Check sheet for the modelled part. Datum: model origin and axes. Units: mm. A direction names the side the tool comes from. Round coordinates to 2 decimals unless told otherwise and drop trailing zeros. Write each loop counter-clockwise with the first axis right and the second up, starting at its lowest first coordinate (ties: lowest second). Pieces come first, ordered by that corner, then holes. Notation, with made-up numbers: M 31,1 L 79,1 A11 cw 79,18 Z; hole C 74.25,79.25 d4. An arc over 180 degrees is marked long. One line per item, written item: value.
from build123d import *

# Parameters (mm, degrees)
SKETCH1_W           = 640
SKETCH1_H           = 50
BOSS_EXTRUDE1_DEPTH = 10
SKETCH2_W           = 15
SKETCH2_H           = 50
BOSS_EXTRUDE2_DEPTH = 10
SKETCH3_W           = 610
SKETCH3_H           = 20
CUT_EXTRUDE1_DEPTH  = 10


with BuildPart() as part:
    # Sketch1 → Boss-Extrude1 (new body)
    with BuildSketch(Plane.XY):
        with Locations((-320, -120.36)):
            Rectangle(SKETCH1_W, SKETCH1_H)
    extrude(amount=BOSS_EXTRUDE1_DEPTH)

    # Sketch2 → Boss-Extrude2 (add)
    with BuildSketch(Plane.XY):
        with Locations((-160, -70.36)):
            Rectangle(SKETCH2_W, SKETCH2_H)
        with Locations((-480, -70.36)):
            Rectangle(SKETCH2_W, SKETCH2_H)
    extrude(amount=BOSS_EXTRUDE2_DEPTH)

    # Sketch3 → Cut-Extrude1 (cut)
    with BuildSketch(Plane(origin=(0, 0, 0), x_dir=(-1, 0, 0), z_dir=(0, 0, -1))):
        with Locations((320, -120.36)):
            Rectangle(SKETCH3_W, SKETCH3_H)
    extrude(amount=-CUT_EXTRUDE1_DEPTH, mode=Mode.SUBTRACT)


solid = part.part
Q1. Draft check along Y on faces 1 (the flat face through (-316, -130.36, 5)), 2 (the flat face through (-167.5, -71, 5)), 3 (the flat face through (-160, -45.36, 5)). Enter one of: pulls with the +Y half, pulls with the -Y half, needs draft (parallel to the pull), parting line crosses it, or undercut.
Completed:
face 1: undercut
face 2: needs draft
face 3: pulls with the +Y half
Q2. Scan lines: line 1 (X direction, y = -70, z = 4.25); line 2 (Y direction, x = -551, z = 7.5); line 3 (X direction, y = -117, z = 8.5). Record each from-to range of solid material in increasing order. Write a range as [from, to].
Completed:
line 1: [-487.5, -472.5], [-167.5, -152.5]
line 2: [-145.36, -130.36], [-110.36, -95.36]
line 3: [-640, -625], [-15, 0]
Q3. Access from +Z, -Z, +X, -X, +Y, -Y to the whole of each face (thin tool, end or side, straight path). Record for faces 4 (the flat face through (-152.5, -71, 5)), 5 (the flat face through (-324, -145.36, 5)), 6 (the flat face through (-565, -95.36, 5)), 7 (the flat face through (-322, -95.36, 5)), 8 (the flat face through (-316, -110.36, 5)).
Completed:
face 4: +Z, -Z, +X, +Y
face 5: +Z, -Z, +X, -X, -Y
face 6: +Z, -Z, -X, +Y
face 7: +Z, -Z, +Y
face 8: +Z, -Z
Q4. Sectioned sample at C-C on z = 4.25. Enter the section's corners in (x, y).
Completed:
outline: M -640,-145.36 L 0,-145.36 L 0,-95.36 L -152.5,-95.36 L -152.5,-45.36 L -167.5,-45.36 L -167.5,-95.36 L -472.5,-95.36 L -472.5,-45.36 L -487.5,-45.36 L -487.5,-95.36 L -640,-95.36 Z; hole M -625,-130.36 L -15,-130.36 L -15,-110.36 L -625,-110.36 Z
Q5. Depth check by flat-ended pin: P1, Ø5, axis at y = -55.5, z = 1.5, coming from the -X side; P2, Ø6, axis at y = -59.5, z = 7, coming from the +X side; P3, Ø3, axis at x = -254.5, z = 6.5, coming from the +Y side. Enter the tip coordinate at first touch or a pass-through.
Completed:
P1: x = -487.5
P2: x = -152.5
P3: y = -95.36
Q6. Sectioned sample at B-B on y = -121.5. Enter the section's corners in (x, z).
Completed:
outline: M -640,0 L -625,0 L -625,10 L -640,10 Z; M -15,0 L 0,0 L 0,10 L -15,10 Z
Q7. Sectioned sample at A-A on x = -459. Enter the section's corners in (y, z), and give its area (3 significant figures).
Completed:
outline: M -145.36,0 L -130.36,0 L -130.36,10 L -145.36,10 Z; M -110.36,0 L -95.36,0 L -95.36,10 L -110.36,10 Z
area: 300 mm^2
